Check sheet for the modelled part. Datum: model origin and axes. Units: mm. A direction names the side the tool comes from. Coordinates: 2 decimals unless noted, no trailing zeros. Loops run counter-clockwise (first coordinate to the right, second up) from the corner with the lowest first, then second, coordinate; pieces in that order, holes last. Notation, with made-up numbers: (62.5, 62) - (101.5, 62) arc R24 ccw to (101.5, 84) - close; hole circle Ø1 at (-20, 24.5). An arc over 180 degrees is marked (long way). Use a Markdown table: item, result. Add a question column.
1) Tool access check on faces 1 (the cylindrical face through (-1.5, -0.07, 8.41)), 2 (the flat face through (0, 0, 15)). Record the directions out of +Z, -Z, +X, -X, +Y, -Y that give a thin tool (end or side, any length) a straight path to the whole face; none if there is none.
2) Sectioned sample at C-C, the plane z = 6.75. Enter the section's corners in (x, y).
3) Thickness scan on line 1 (Y direction, x = -0.1, z = 12); line 2 (Z direction, x = -0.65, y = -1.95); line 3 (Z direction, x = 2.4, y = -0.5). Record the ranges inside material, lowest first.
4) Go/stop test with flat-tipped pins: P1, Ø3, axis at x = 0.5, z = 8, coming from the +Y side; P2, Ø1.5, axis at x = -1, z = 8.5, coming from the -Y side. Record where each tip stops, or that it passes through.
Autodesk Inventor part; units mm, degrees
ref_plane "YZ Plane" through (0, 0, 0) normal (1, 0, 0) x (0, 1, 0)
ref_plane "XZ Plane" through (0, 0, 0) normal (0, 1, 0) x (-1, 0, 0)
ref_plane "XY Plane" through (0, 0, 0) normal (0, 0, 1) x (1, 0, 0)
sketch "スケッチ1" plane through (0, 0, 0) normal (0, 0, 1) x (1, 0, 0)
  circle A0 centre (0, 0) radius 1.5
  dimension "d0" = 3
extrude "押し出し1" add sketch "スケッチ1" along normal blind 15
sketch "スケッチ2" plane through (0, 0, 0) normal (0, 0, -1) x (-1, 0, 0)
  circle A0 centre (0, 0) radius 3
  dimension "d3" = 6
extrude "押し出し2" add sketch "スケッチ2" against normal blind 2
thread "ねじ1"
chamfer "面取り1" distance 1.5 angle 45 1 edges at (3, 0, 2)
properties part number "ネジ皿m3,15" material "鋼、高強度、低合金"
Solved:
| question | item | result |
|---|---|---|
| 1 | face 1 | +Z |
| 1 | face 2 | +Z, +X, -X, +Y, -Y |
| 2 | outline | circle Ø3 at (0, 0) |
| 3 | line 1 | y = -1.5 to 1.5 |
| 3 | line 2 | z = 0 to 1.44 |
| 3 | line 3 | z = 0 to 1.05 |
| 4 | P1 | stops at y = 1.5 |
| 4 | P2 | stops at y = -1.48 |
